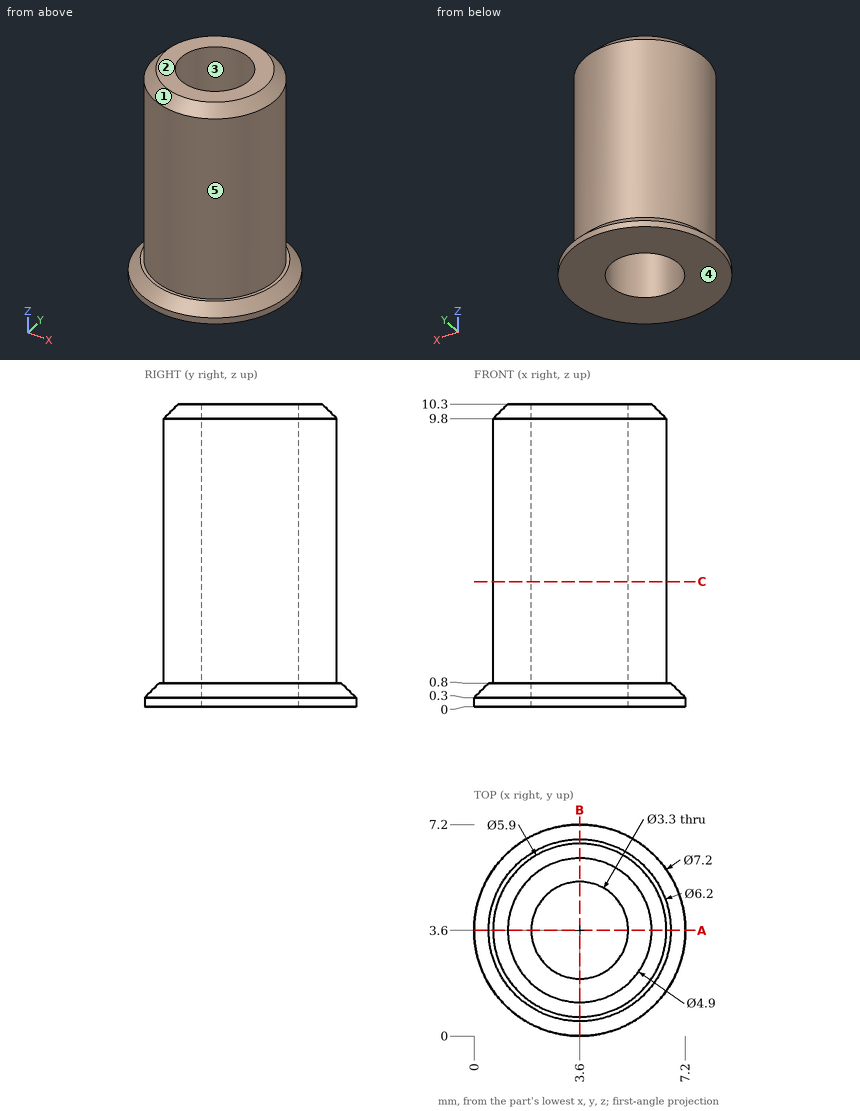
For this review, use the dimensioned drawing (mm, ordinates from the lowest corner) and the shaded views. A direction names the side the tool comes from. Round coordinates to 2 decimals unless told otherwise and drop trailing zeros. Write each loop counter-clockwise with the first axis right and the second up, starting at its lowest first coordinate (ties: lowest second). Pieces come first, ordered by that corner, then holes. Notation, with made-up numbers: (-18, 77.25) -> (-10, 77.25) arc R26 ccw to (-10, 102.25) -> close; hole circle Ø7 at (24.25, -35.5). An arc over 180 degrees is marked (long way). One line per item, written item: value. Start each with the question number.
Q1. Add section A-A (y = 3.6). Give the boundary of the cut face in (x, z), then the cut area to 3 significant figures.
Q2. Add section C-C (z = 4.25). Give the boundary of the cut face in (x, y), then the cut area to 3 significant figures.
Q3. To check wall thickness, follow probe 1 along Y at (x, z) = (3.6, 3.75); probe 2 along Y at (x, z) = (4.5, 1.5); probe 3 along X at (y, z) = (4.75, 8). State the ranges of each line that lie inside material, in increasing order.
Q4. Insertion check: P1, Ø1, axis at x = 5, z = 2.5, coming from the -Y side; P2, Ø1, axis at y = 2, z = 5, coming from the -X side; P3, Ø2, axis at x = 2, y = 3.5, coming from the +Z side. Each pin has a flat end and moves straight along its axis. Give the tip position at first contact, or say it passes through.
Q5. The part is to be moulded in two halves that separate along X. For the marked faces 1, 2 and 3, say which applies: pulls with the +X half, pulls with the -X half, needs draft (parallel to the pull), parting line crosses it, or undercut.
Q6. Tool access review of the marked faces 4 and 5: name each direction out of +Z, -Z, +X, -X, +Y, -Y from which nothing blocks a thin tool from reaching the whole face with its end or side.
Response:
1. outline: (0, 0) -> (1.95, 0) -> (1.95, 10.3) -> (1.15, 10.3) -> (0.65, 9.8) -> (0.65, 0.8) -> (0.5, 0.8) -> (0, 0.3) -> close; (5.25, 0) -> (7.2, 0) -> (7.2, 0.3) -> (6.7, 0.8) -> (6.55, 0.8) -> (6.55, 9.8) -> (6.05, 10.3) -> (5.25, 10.3) -> close
1. area: 27.3 mm^2
2. outline: circle Ø5.9 at (3.6, 3.6); hole circle Ø3.3 at (3.6, 3.6)
2. area: 18.8 mm^2
3. probe 1: y = 0.65 to 1.95, 5.25 to 6.55
3. probe 2: y = 0.79 to 2.22, 4.98 to 6.41
3. probe 3: x = 0.88 to 2.42, 4.78 to 6.32
4. P1: stops at y = 0.79
4. P2: stops at x = 0.86
4. P3: stops at z = 10.3
5. face 1: parting line crosses it
5. face 2: needs draft
5. face 3: undercut
6. face 4: -Z, +X, -X, +Y, -Y
6. face 5: +Z
